The listing builds one solid part. Answer for the finished solid, in the listing's coordinates (mm). A direction names the side the tool comes from. Give positions to 0.01 mm unless a question says otherwise; leave off trailing zeros. Order: outer loops, then holes, each group sorted by start corner. A loop starts at its lowest first (then second) coordinate and runs counter-clockwise, first axis right, second up. Notation, with made-up numbers: (-32, 53) - (19, 53) arc R31 ccw to (19, 92) - close; hole circle Ø8 at (-25, 3). An arc over 180 degrees is marked (long way). Answer as a JSON object with one key per item and string values. Group by question number.
Q1. Given pin 1 (1.5 mm diameter, centred on x = -30, y = -17.5, fed in from -Z) (3 decimals); pin 2 (10 mm diameter, centred on x = -76.5, z = 18.5, fed in from +Y); pin 3 (8.5 mm diameter, centred on y = -1.5, z = 15, fed in from -X); pin 4 (7.5 mm diameter, centred on x = -99.5, z = 8, fed in from +Y), each flat-ended and moving along its own axis, determine where each tip first touches the part or whether it passes through.
Q2. For faces 5 (the face through (-83.348, -1, 13)), 6 (the face through (-11, 16.618, 13)), 7 (the face through (-30, 0, 0)), 8 (the face through (-13, -15.995, 13)), determine the directions among +Z, -Z, +X, -X, +Y, -Y from which every point of the face is accessible in a straight line to the end or side of a thin tool.
Q3. A cutting plane is placed at A-A, the plane x = -89. Give the vertices of the cut face in (y, z).
Q4. The mould has two halves that part along Y. Classify faces 1 (the face through (-103, -9.249, 13)), 2 (the face through (59.091, -11.422, 12.522)), 3 (the face through (-103, 7.846, 13)), 4 (the face through (-104.57, 25.58, 12.52)): released by +Y, released by -Y, zero draft, split by the parting line, or undercut.
Q5. A cutting plane is placed at C-C, the plane x = -24. Give the vertices of the cut face in (y, z), and give its area (3 significant figures).
Q6. A cutting plane is placed at B-B, the plane z = 14.75. Give the vertices of the cut face in (x, y).
Q7. A cutting plane is placed at D-D, the plane y = 22. Give the vertices of the cut face in (x, z).
Q8. Consider line 1 (X direction, y = 0, z = 15.5); line 2 (Y direction, x = -42, z = 10.25); line 3 (Y direction, x = -83.5, z = 1.25). Determine where each line is inside the solid, lowest interval first.
from build123d import *

# Parameters (mm, degrees)
F1_DEPTH    = 25.4
F3_DEPTH    = 38.1
F4_R        = 12.7
F5_R        = 12.7
F6_T1_DEPTH = 114.3


# Not quite as in the source:
# - a fillet or chamfer that OpenCascade refuses, or shapes differently, is made with other operations: its cross-section is extruded or revolved along the edge and cut away or added


with BuildPart() as f1:
    # F0 (on Top) → F1 (new body)
    with BuildSketch(Plane.XY):
        with BuildLine():
            Line((-77.2201499837, 16.618498601), (-92.2268889844, 16.618498601))
            Line((-92.2268889844, 16.618498601), (-92.2268889844, -15.9945080916))
            Line((-92.2268889844, -15.9945080916), (-76.7317300981, -15.9945080916))
            ThreePointArc((-76.7317300981, -15.9945080916), (-72.7314875025, -8.4378237077), (-71.3499844152, 0))
            ThreePointArc((-71.3499844152, 0), (-72.8606518933, 8.8123966597), (-77.2201499837, 16.618498601))
        make_face()
        with BuildLine():
            Line((64.9677813053, 16.618498601), (-77.2201499837, 16.618498601))
            ThreePointArc((-77.2201499837, 16.618498601), (-72.8606518933, 8.8123966597), (-71.3499844152, 0))
            ThreePointArc((-71.3499844152, 0), (-72.7314875025, -8.4378237077), (-76.7317300981, -15.9945080916))
            Line((-76.7317300981, -15.9945080916), (64.9677813053, -15.9945080916))
            Line((64.9677813053, -15.9945080916), (64.9677813053, 16.618498601))
        make_face()
        with BuildLine():
            Line((-92.2268889844, -15.9945080916), (-92.2268889844, 16.618498601))
            Line((-92.2268889844, 16.618498601), (-77.2201499837, 16.618498601))
            ThreePointArc((-77.2201499837, 16.618498601), (-124.2643223617, -0.3962064299), (-76.7317300981, -15.9945080916))
            Line((-76.7317300981, -15.9945080916), (-92.2268889844, -15.9945080916))
        make_face()
    extrude(amount=F1_DEPTH)

    # F2 (on face) → F3 (cut)
    with BuildSketch(Plane.XY.offset(25.4)):
        with BuildLine():
            Line((-83.348184824, 7.8462203965), (-123.0771370274, 7.8462203965))
            ThreePointArc((-123.0771370274, 7.8462203965), (-124.2569046236, -0.741220082), (-122.5980357113, -9.2491069809))
            Line((-122.5980357113, -9.2491069809), (-83.348184824, -9.2491069809))
            Line((-83.348184824, -9.2491069809), (-83.348184824, 7.8462203965))
        make_face()
        with BuildLine():
            Line((-123.0771370274, 7.8462203965), (-131.8430900574, 7.8462203965))
            Line((-131.8430900574, 7.8462203965), (-131.8430900574, -9.2491069809))
            Line((-131.8430900574, -9.2491069809), (-122.5980357113, -9.2491069809))
            ThreePointArc((-122.5980357113, -9.2491069809), (-124.2569046236, -0.741220082), (-123.0771370274, 7.8462203965))
        make_face()
    extrude(amount=-F3_DEPTH, mode=Mode.SUBTRACT)

    # F4
    f4_edges = [f1.edges().sort_by_distance(p)[0] for p in [
        (-77.22015, 16.618499, 12.7),
    ]]
    fillet(f4_edges, radius=F4_R)

    # F5
    f5_edges = [f1.edges().sort_by_distance(p)[0] for p in [
        (-76.73173, -15.994508, 12.7),
    ]]
    fillet(f5_edges, radius=F5_R)

    # F6: fillet of radius 17.78 on 2 edges, made by hand

    # F6_s2 → F6_t1 (cut)
    with BuildSketch(Plane.XY.offset(-44.45)):
        with BuildLine():
            ThreePointArc((64.9677813053, -1.161501399), (59.7601398748, 11.4108571705), (47.1877813053, 16.618498601))
            Line((47.1877813053, 16.618498601), (64.9677813053, 16.618498601))
            Line((64.9677813053, 16.618498601), (64.9677813053, -1.161501399))
        make_face()
        with BuildLine():
            ThreePointArc((47.1877813053, -15.9945080916), (59.7601398748, -10.7868666611), (64.9677813053, 1.7854919084))
            Line((64.9677813053, 1.7854919084), (64.9677813053, -15.9945080916))
            Line((64.9677813053, -15.9945080916), (47.1877813053, -15.9945080916))
        make_face()
    extrude(amount=F6_T1_DEPTH, mode=Mode.SUBTRACT)


solid = f1.part
Reply:
{
 "1": {"pin 1": "passes through", "pin 2": "stops at y = 20.83", "pin 3": "stops at x = -83.35", "pin 4": "stops at y = 26.46"},
 "2": {"face 5": "+Z, -Z, -X", "face 6": "+Z, -Z, +X, +Y", "face 7": "-Z, +X, -X, +Y, -Y", "face 8": "+Z, -Z, +X, -Y"},
 "3": {"outline": "(-24.95, 0) - (-9.25, 0) - (-9.25, 25.4) - (-24.95, 25.4) - close; (7.85, 0) - (24.95, 0) - (24.95, 25.4) - (7.85, 25.4) - close"},
 "4": {"face 1": "undercut", "face 2": "released by -Y", "face 3": "undercut", "face 4": "released by +Y"},
 "5": {"outline": "(-15.99, 0) - (16.62, 0) - (16.62, 25.4) - (-15.99, 25.4) - close", "area": "828 mm^2"},
 "6": {"outline": "(-123.08, 7.85) - (-83.35, 7.85) - (-83.35, -9.25) - (-122.6, -9.25) arc R26.46 ccw to (-79.8, -19.39) arc R12.7 cw to (-71.16, -15.99) - (47.19, -15.99) arc R17.78 ccw to (64.91, 0.31) arc R17.78 ccw to (47.19, 16.62) - (-71.85, 16.62) arc R12.7 cw to (-80.27, 19.81) arc R26.46 ccw to start"},
 "7": {"outline": "(-112.51, 0) - (-83.11, 0) - (-83.11, 25.4) - (-112.51, 25.4) - close"},
 "8": {"line 1": "x = -83.35 to 64.88", "line 2": "y = -15.99 to 16.62", "line 3": "y = -22.26 to -9.25, 7.85 to 22.26"}
}
